Model file for the job. Use its own axes, mm. Face numbers are marked on the shaded views. A direction names the side the tool comes from. Coordinates: 2 decimals unless noted, no trailing zeros. Loops run counter-clockwise (first coordinate to the right, second up) from the corner with the lowest first, then second, coordinate; pieces in that order, holes last. Notation, with made-up numbers: M 43.5,61 L 63.5,61 A24 ccw 63.5,78 Z; hole C -11.5,-18 d1. An arc over 180 degrees is marked long. One line per question, with ' | ' between items. Start each with the question number.
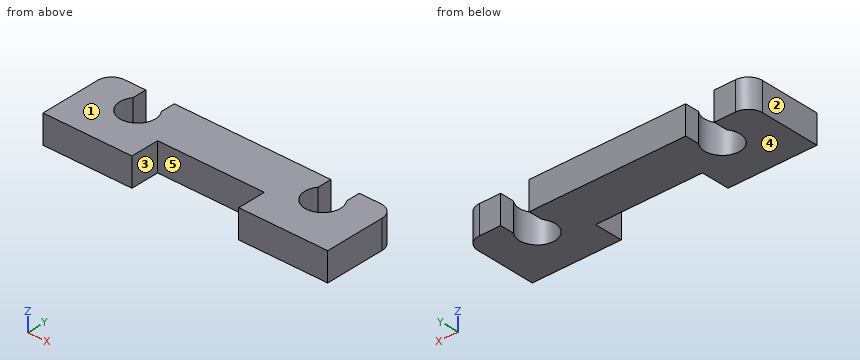
```python
from build123d import *

# Parameters (mm, degrees)
TUBE_PLATE_BODY_DEPTH   = 2
TUBE_PLATE_CONTOURING_R = 1


with BuildPart() as part:
    # Sketch1 → Tube Plate Body (new body)
    with BuildSketch(Plane.XY):
        with BuildLine():
            Line((-10, 0), (-10, 5.25))
            Line((-10, 5.25), (-7.5, 5.25))
            Line((-7.5, 5.25), (-7.5, 4.25))
            ThreePointArc((-7.5, 4.25), (-6.5, 2.25), (-5.5, 4.25))
            Line((-5.5, 4.25), (-5.5, 5.25))
            Line((-5.5, 5.25), (5.5, 5.25))
            Line((5.5, 5.25), (5.5, 4.25))
            ThreePointArc((5.5, 4.25), (6.5, 2.25), (7.5, 4.25))
            Line((7.5, 4.25), (7.5, 5.25))
            Line((7.5, 5.25), (10, 5.25))
            Line((10, 5.25), (10, 0))
            Line((10, 0), (3.75, 0))
            Line((3.75, 0), (3.75, 2))
            Line((3.75, 2), (-3.75, 2))
            Line((-3.75, 2), (-3.75, 0))
            Line((-3.75, 0), (-10, 0))
        make_face()
    extrude(amount=TUBE_PLATE_BODY_DEPTH)

    # Tube Plate Contouring
    tube_plate_contouring_edges = [part.edges().sort_by_distance(p)[0] for p in [
        (-10, 5.25, 1),
        (10, 5.25, 1),
    ]]
    fillet(tube_plate_contouring_edges, radius=TUBE_PLATE_CONTOURING_R)


solid = part.part
```
(1) Band-saw the part on B-B on y = 3.5. Write the cut outline in (x, z).
(2) 3-axis set-ups, long thin cutter, end or side, ignore diameter. For the marked faces 4 and 5: which of +Z, -Z, +X, -X, +Y, -Y reach the whole face in a straight line?
(3) Pin check, flat tips, straight feed: P1, Ø1.1, axis at y = 5, z = 1.5, coming from the +X side; P2, Ø2, axis at x = -6.5, y = 3.5, coming from the -Z side (1 decimal); P3, Ø0.5, axis at y = 5, z = 0.5, coming from the -X side; P4, Ø0.6, axis at x = 0, z = 1, coming from the -Y side. Stop position of each tip, or through.
(4) Band-saw the part on C-C on z = 0.7. Write the cut outline in (x, y).
(5) Drill centre lines: line 1 (X direction, y = 3.5, z = 1); line 2 (X direction, y = 2.75, z = 1.95); line 3 (X direction, y = 1.65, z = 1.8). Where is each one in solid material? Low to high. Write a range as [from, to].
(6) Two-plate mould, pull along X, no slides. Class the marked faces 1, 2 and 3: pulls with the +X half, pulls with the -X half, needs draft (parallel to the pull), parting line crosses it, or undercut.
(7) Band-saw the part on D-D on x = -6.5. Write the cut outline in (y, z), then the cut area to 3 significant figures.
(8) Band-saw the part on A-A on y = 1.1. Write the cut outline in (x, z).
Computed values:
1) outline: M -10,0 L -7.75,0 L -7.75,2 L -10,2 Z; M -5.25,0 L 5.25,0 L 5.25,2 L -5.25,2 Z; M 7.75,0 L 10,0 L 10,2 L 7.75,2 Z
2) face 4: -Z, +X, -X, +Y, -Y | face 5: +Z, -Z, -Y
3) P1: x = 9.98 | P2: through | P3: x = -9.87 | P4: y = 2
4) outline: M -10,0 L -3.75,0 L -3.75,2 L 3.75,2 L 3.75,0 L 10,0 L 10,4.25 A1 ccw 9,5.25 L 7.5,5.25 L 7.5,4.25 A1.25 cw long 5.5,4.25 L 5.5,5.25 L -5.5,5.25 L -5.5,4.25 A1.25 cw long -7.5,4.25 L -7.5,5.25 L -9,5.25 A1 ccw -10,4.25 Z
5) line 1: [-10, -7.75], [-5.25, 5.25], [7.75, 10] | line 2: [-10, -7.5], [-5.5, 5.5], [7.5, 10] | line 3: [-10, -3.75], [3.75, 10]
6) face 1: needs draft | face 2: pulls with the -X half | face 3: undercut
7) outline: M 0,0 L 2.25,0 L 2.25,2 L 0,2 Z | area: 4.50 mm^2
8) outline: M -10,0 L -3.75,0 L -3.75,2 L -10,2 Z; M 3.75,0 L 10,0 L 10,2 L 3.75,2 Z
